For this review, take the finished solid that the model builds, in its own axes (mm). Give positions to 0.01 mm unless a question says otherwise; leave off trailing zeros. Loops run counter-clockwise (first coordinate to the right, second up) from the corner with the lowest first, then second, coordinate; pieces in that order, holes last.
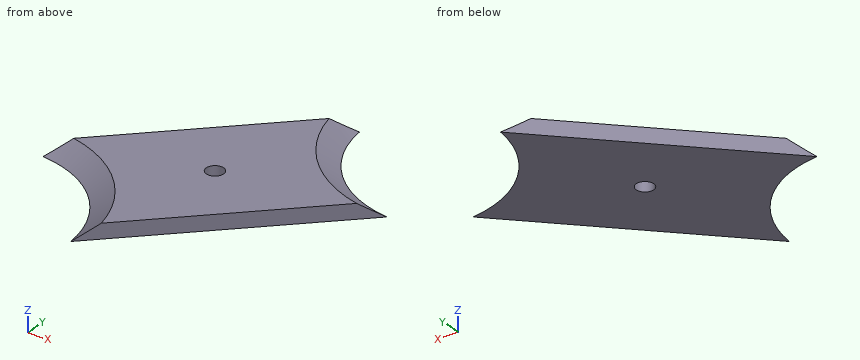
```python
from build123d import *

# Parameters (mm, degrees)
SKETCH3_R           = 2.94685624
BOSS_EXTRUDE1_DEPTH = 5
CHAMFER1_SIZE2      = 6.881909602
CHAMFER1_SIZE       = 5
CHAMFER2_SIZE2      = 5
CHAMFER2_SIZE       = 6.881909602


with BuildPart() as part:
    # Sketch3 → Boss-Extrude1 (new body)
    with BuildSketch(Plane.XY):
        with BuildLine():
            Line((48.567273068, 137.828283654), (110.567273068, 199.828283654))
            ThreePointArc((110.567273068, 199.828283654), (121.583561944, 176.84457253), (144.567273068, 165.828283654))
            Line((144.567273068, 165.828283654), (82.567273068, 103.828283654))
            ThreePointArc((82.567273068, 103.828283654), (71.734296399, 126.995306985), (48.567273068, 137.828283654))
        make_face()
        with Locations((96.567273068, 151.828283654)):
            Circle(SKETCH3_R, mode=Mode.SUBTRACT)
    extrude(amount=BOSS_EXTRUDE1_DEPTH)

    # Chamfer1
    chamfer1_edges = [part.edges().sort_by_distance(p)[0] for p in [
        (121.583561944, 176.84457253, 5),
    ]]
    chamfer1_side = [part.faces().sort_by_distance(p)[0] for p in [
        (121.583561944, 176.84457253, 4.9),
    ]]
    chamfer(chamfer1_edges, length=CHAMFER1_SIZE - 0.0001, length2=CHAMFER1_SIZE2 - 0.0001, reference=chamfer1_side[0])  # a hair under: the kernel refuses the full size

    # Chamfer2
    chamfer2_edges = [part.edges().sort_by_distance(p)[0] for p in [
        (71.734296399, 126.995306985, 5),
    ]]
    chamfer2_side = [part.faces().sort_by_distance(p)[0] for p in [
        (71.805007077, 127.066017663, 5),
    ]]
    chamfer(chamfer2_edges, length=CHAMFER2_SIZE - 0.0001, length2=CHAMFER2_SIZE2 - 0.0001, reference=chamfer2_side[0])  # a hair under: the kernel refuses the full size


solid = part.part
```
Item 1: Take a section at B-B on z = 0.9. Give the boundary of the cut face in (x, y).
Answer:
outline: (49.7, 138.96) arc R38.74 cw to (83.7, 104.96) - (143.45, 164.72) arc R39.62 cw to (109.45, 198.72) - close; hole circle Ø5.89 at (96.57, 151.83)
Item 2: Clearance check with flat-ended pins moving along their axes: pin 1 Ø2 at (y, z) = (167, 3.5) entering from -X; pin 2 Ø3 at (x, z) = (78, 2.5) entering from +Y. State where each tip first meets the part, or that it passes through.
Answer:
pin 1: stops at x = 76.74
pin 2: stops at y = 168.76
Item 3: Take a section at A-A on x = 96.5. Give the boundary of the cut face in (y, z), and give its area (3 significant figures).
Answer:
outline: (117.76, 0) - (148.88, 0) - (148.88, 5) - (117.76, 5) - close; (154.77, 0) - (185.76, 0) - (185.76, 5) - (154.77, 5) - close
area: 311 mm2
Item 4: For L1, parallel to Y at x = 94.5, z = 4.3; L2, parallel to Y at x = 96, z = 4.3; L3, parallel to X at y = 171.5, z = 1.35, list the stretches that pass through material, from the lowest coordinate up.
Answer:
L1: y = 115.76 to 149.73, 153.93 to 183.76
L2: y = 117.26 to 148.94, 154.72 to 185.26
L3: x = 82.24 to 124.98
